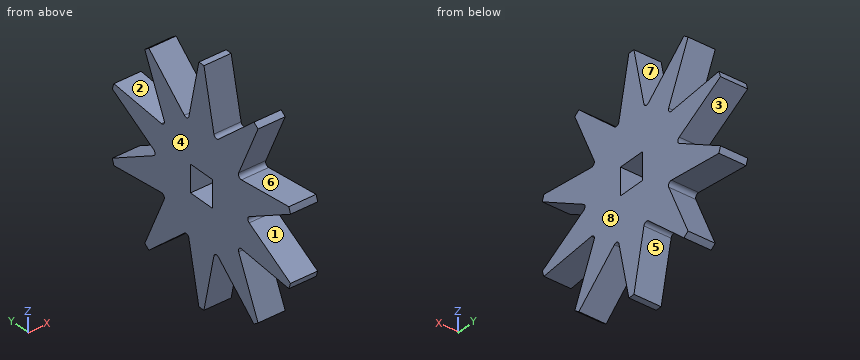
Autodesk Inventor part; units mm, degrees
ref_plane "YZ Plane" through (0, 0, 0) normal (1, 0, 0) x (0, 1, 0)
ref_plane "XZ Plane" through (0, 0, 0) normal (0, 1, 0) x (-1, 0, 0)
ref_plane "XY Plane" through (0, 0, 0) normal (0, 0, 1) x (1, 0, 0)
sketch "Sketch1" plane through (0, 0, 0) normal (1, 0, 0) x (0, 1, 0)
  circle A0 centre (0, 0) radius 53.975
  line L0 (-6.35, 6.35) -> (6.35, 6.35)
  line L1 (6.35, 6.35) -> (6.35, -6.35)
  line L2 (6.35, -6.35) -> (-6.35, -6.35)
  line L3 (-6.35, -6.35) -> (-6.35, 6.35)
  line L4 (-6.35, 6.35) -> (0, 0) construction
  line L5 (0, 0) -> (6.35, 6.35) construction
  line L6 (-6.35, -6.35) -> (0, 0) construction
  line L7 (0, 0) -> (6.35, -6.35) construction
  dimension "d0" = 107.95
  dimension "d1" = 12.7
extrude "Extrusion1" add sketch "Sketch1" along normal blind 12.7
sketch "Sketch2" plane through (12.7, 0, 0) normal (1, 0, 0) x (0, 0, -1)
  circle A0 centre (0, 0) radius 53.975
  line L0 (0, 0) -> (0, 53.975) construction
  line L1 (0, 53.975) -> (-15.2606, 51.7727) construction
  line L2 (0, 53.975) -> (15.2606, 51.7727) construction
  line L3 (15.2606, 51.7727) -> (0, 0) construction
  line L4 (0, 0) -> (-15.2606, 51.7727) construction
  arc A1 (15.2606, 51.7727) -> (-15.2606, 51.7727) centre (0, 0) ccw construction
  line L5 (-15.2606, 51.7727) -> (-1.374, 27.7798)
  line L6 (1.374, 27.7798) -> (15.2606, 51.7727)
  arc A2 (-1.374, 27.7798) -> (1.374, 27.7798) centre (0, 28.575) ccw
  dimension "d4" = 32.847
  dimension "d11" = 1.5875
  dimension "d12" = 25.4
extrude "Extrusion3" cut sketch "Sketch2" against normal through all contours L6 A2 L5 A0 picked at (-7.2613, 44.4271)
pattern_circular "Circular Pattern2" count 10 over 360 about axis through (0, 0, 0) along (1, 0, 0) of "Extrusion3"
properties part number "IntakeRoller" material "Silicone"
The listing builds one solid part. Answer for the finished solid, in the listing's coordinates (mm). Face numbers are marked on the shaded views. A direction names the side the tool comes from. Give positions to 0.01 mm unless a question says otherwise; leave off trailing zeros. Write each loop counter-clockwise with the first axis right and the second up, starting at its lowest first coordinate (ties: lowest second). Pieces come first, ordered by that corner, then holes. Notation, with made-up numbers: (52, 29) - (93, 29) arc R8 ccw to (93, 43) - close; hole circle Ø10 at (81, 42.5). An arc over 180 degrees is marked (long way). Use a Markdown table: item, result.
1. Section A-A on y = 42 is taken. Write down the section's boundary in (x, z).
Values follow:
| item | result |
|---|---|
| outline | (0, -17.16) - (12.7, -17.16) - (12.7, -9.6) - (0, -9.6) - close; (0, 9.6) - (12.7, 9.6) - (12.7, 17.16) - (0, 17.16) - close |
2. Section C-C on z = -39.5 is taken. Write down the section's boundary in (x, y).
Values follow:
| item | result |
|---|---|
| outline | (0, -31.46) - (12.7, -31.46) - (12.7, -24.92) - (0, -24.92) - close; (0, -4.57) - (12.7, -4.57) - (12.7, 4.57) - (0, 4.57) - close; (0, 24.92) - (12.7, 24.92) - (12.7, 31.46) - (0, 31.46) - close |
3. Section D-D on y = -15 is taken. Write down the section's boundary in (x, z).
Values follow:
| item | result |
|---|---|
| outline | (0, -30.59) - (12.7, -30.59) - (12.7, 30.59) - (0, 30.59) - close |
4. Each of these flat-tipped pins is pushed along its axis until it touches: P1, Ø4, axis at x = 10.5, z = -20, coming from the +Y side; P2, Ø4, axis at x = 8, z = 0.5, coming from the +Y side; P3, Ø3, axis at x = 4.5, y = 40, coming from the -Z side. Where does it stop, or does it pass through?
Values follow:
| item | result |
|---|---|
| P1 | stops at y = 50.89 |
| P2 | stops at y = 29.73 |
| P3 | stops at z = -17.11 |
5. Section B-B on z = -4 is taken. Write down the section's boundary in (x, y), plus the area to 3 significant figures.
Values follow:
| item | result |
|---|---|
| outline | (0, -32.32) - (12.7, -32.32) - (12.7, -6.35) - (0, -6.35) - close; (0, 6.35) - (12.7, 6.35) - (12.7, 32.32) - (0, 32.32) - close |
| area | 660 mm² |
6. For a pull along Y with two mould halves and no side action, classify the marked faces 1, 2 and 3 as released by +Y, released by -Y, zero draft, split by the parting line, or undercut.
Values follow:
| item | result |
|---|---|
| face 1 | released by -Y |
| face 2 | undercut |
| face 3 | released by +Y |
7. Find the intervals of material crossed by probe 1 along Z at (x, y) = (5.5, 1); probe 2 along Y at (x, z) = (6, 42.5); probe 3 along Z at (x, y) = (8.5, 24), in increasing order. Write a range as from..to.
Values follow:
| item | result |
|---|---|
| probe 1 | z = -53.97..-6.35, 6.35..53.97 |
| probe 2 | y = -32.79..-28.26, -3.93..3.93, 28.26..32.79 |
| probe 3 | z = -38.67..-22.7, -15.29..15.29, 22.7..38.67 |
8. A tool of negligible diameter and unlimited length cuts with its end or side. For the marked faces 4, 5, 6, 7 and 8, from which of +Z, -Z, +X, -X, +Y, -Y can it reach the whole face along a straight path? Write none if from no direction.
Values follow:
| item | result |
|---|---|
| face 4 | +Z, -Z, -X, +Y, -Y |
| face 5 | -Z, +X, -X |
| face 6 | +X, -X |
| face 7 | +Z, +X, -X |
| face 8 | +Z, -Z, +X, +Y, -Y |
